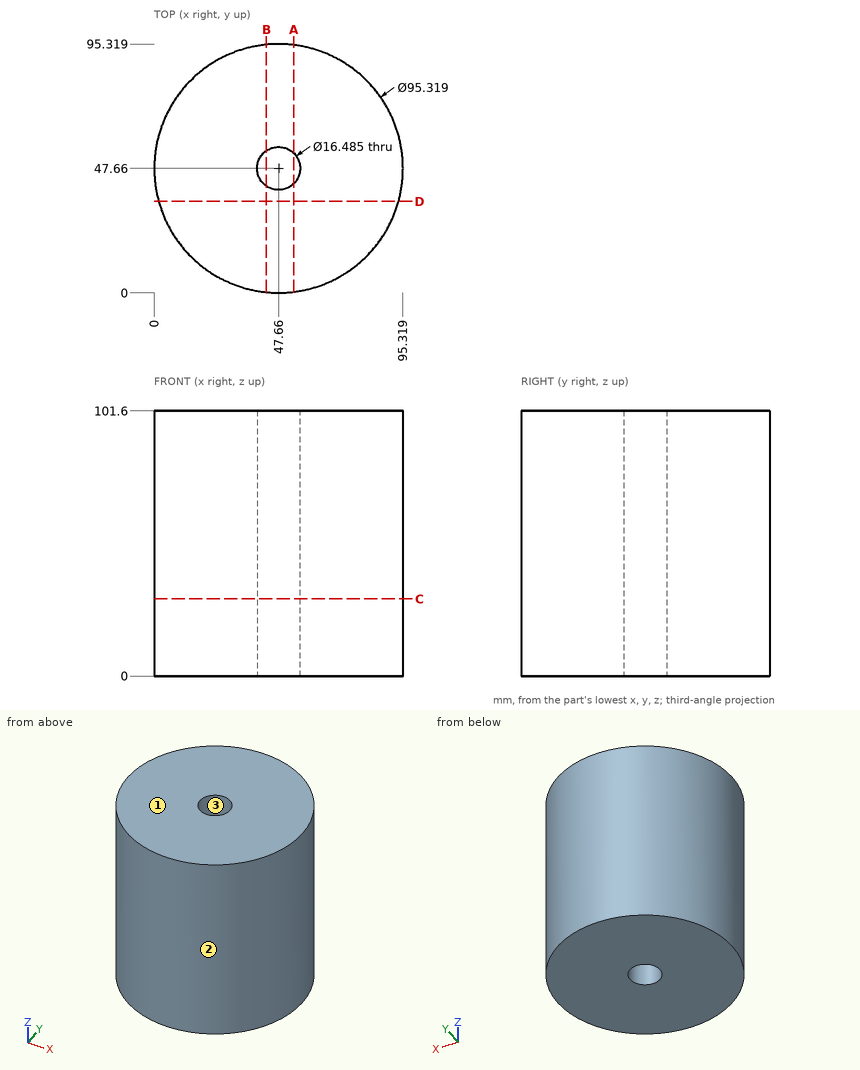
Print and shaded views of the part. All mm, measured from the part's lowest x, y and z. Round coordinates to 2 decimals unless told otherwise and drop trailing zeros. Write each loop counter-clockwise with the first axis right and the second up, starting at its lowest first coordinate (ties: lowest second). Pieces come first, ordered by that corner, then holes. Notation, with made-up numbers: M 28.5,-19 L 64.5,-19 A28 ccw 64.5,9 Z; hole C -23,61.5 d8. An arc over 180 degrees is marked long. Use a Markdown table: item, result. Add a question column.
1. Flat gauge pins, fed straight in: P1, Ø6, axis at x = 30.5, z = 65.5, coming from the +Y side; P2, Ø1, axis at y = 59, z = 74.5, coming from the +X side; P3, Ø2, axis at y = 68, z = 74.5, coming from the +X side; P4, Ø21.5, axis at x = 47.66, y = 47.66, coming from the +Z side. Where does each tip first touch, or does it go through?
2. Slice it at C-C on z = 29.5. Give the cut face in (x, y) (1 decimal).
3. Slice it at B-B on x = 43. Give the cut face in (y, z).
4. Pull direction X, two halves, no side cores. Call the marked faces 1, 2 and 3: released by +X, released by -X, zero draft, split by the parting line, or undercut.
5. Slice it at A-A on x = 53.5. Give the cut face in (y, z) (1 decimal), then the cut area to 3 significant figures.
6. Slice it at D-D on y = 35. Give the cut face in (x, z).
7. Drill centre lines: probe 1 along X at (y, z) = (48, 15) (1 decimal); probe 2 along X at (y, z) = (53, 75.5); probe 3 along Y at (x, z) = (12, 74). Where is each one in solid material? Low to high.
Reply:
| question | item | result |
|---|---|---|
| 1 | P1 | stops at y = 93.17 |
| 1 | P2 | stops at x = 94.07 |
| 1 | P3 | stops at x = 91.22 |
| 1 | P4 | stops at z = 101.6 |
| 2 | outline | C 47.7,47.7 d95.3; hole C 47.7,47.7 d16.5 |
| 3 | outline | M 0.23,0 L 40.86,0 L 40.86,101.6 L 0.23,101.6 Z; M 54.46,0 L 95.09,0 L 95.09,101.6 L 54.46,101.6 Z |
| 4 | face 1 | zero draft |
| 4 | face 2 | split by the parting line |
| 4 | face 3 | undercut |
| 5 | outline | M 0.4,0 L 41.8,0 L 41.8,101.6 L 0.4,101.6 Z; M 53.5,0 L 95,0 L 95,101.6 L 53.5,101.6 Z |
| 5 | area | 8,430 mm^2 |
| 6 | outline | M 1.71,0 L 93.61,0 L 93.61,101.6 L 1.71,101.6 Z |
| 7 | probe 1 | x = 0 to 39.4, 55.9 to 95.3 |
| 7 | probe 2 | x = 0.3 to 41.38, 53.94 to 95.02 |
| 7 | probe 3 | y = 16.04 to 79.28 |
